Solid Edge part; units mm, degrees
sketch "Sketch1" plane through (0, 0, 0) normal (0, 0, 1) x (1, 0, 0)
  line L0 (-42.5, -23) -> (42.5, -23)
  line L1 (42.5, -23) -> (42.5, 23)
  line L2 (42.5, 23) -> (-42.5, 23)
  line L3 (-42.5, 23) -> (-42.5, -23)
  dimension "D1" = 42.5
  dimension "D2" = 42.5
extrude "Protrusion1" add sketch "Sketch1" along normal mid plane 27
sketch "Sketch2" plane through (0, 0, -13.5) normal (0, 0, -1) x (0, 1, 0)
  line L0 (-0.89, 32.61) -> (17.11, 32.61)
  line L1 (17.11, 32.61) -> (17.11, -22.39)
  line L2 (17.11, -22.39) -> (-0.89, -22.39)
  line L3 (-0.89, -22.39) -> (-0.89, 32.61)
extrude "Extrusionsausprägung_2" add sketch "Sketch2" along normal blind 4
sketch "Sketch3" plane through (0, 0, 13.5) normal (0, 0, 1) x (0, 1, 0)
  line L0 (23, -5.61) -> (23, 5.89)
  line L1 (23, 5.89) -> (21.29, 5.89)
  line L2 (21.29, 5.89) -> (21.29, 7.39)
  line L3 (21.29, 7.39) -> (16.29, 7.39)
  line L4 (16.29, 7.39) -> (16.29, 22.89)
  line L5 (16.29, 22.89) -> (2.29, 22.89)
  line L6 (2.29, 22.89) -> (2.29, 14.39)
  line L7 (2.29, 14.39) -> (-9.29, 14.39)
  line L8 (-9.29, 14.39) -> (-16.29, 7.39)
  line L9 (-21.29, 7.39) -> (-16.29, 7.39)
  line L10 (-21.29, 5.89) -> (-21.29, 7.39)
  line L11 (-23, 5.89) -> (-21.29, 5.89)
  line L12 (-23, -5.61) -> (-23, 5.89)
  dimension "D1" = 21.29
  dimension "D2" = 16.29
revolve "RevolvedCutout1" cut sketch "Sketch3" angle 360 about axis through (5.61, -23, 13.5) along (0, 1, 0)
sketch "Sketch4" plane through (-24.195, 0, 13.5) normal (0, 0, 1) x (1, 0, 0)
  line L0 (-5.355, 12) -> (-0.255, 12)
  line L1 (-0.255, 0) -> (-0.255, 12)
  line L2 (-5.355, 0) -> (-0.255, 0)
  line L3 (-5.355, 12) -> (-5.355, 0)
  dimension "D1" = 5.355
revolve "RevolvedCutout2" cut sketch "Sketch4" angle 360 about axis through (0, 0, 13.5) along (1, 0, 0)
sketch "Sketch5" plane through (-24.195, 0, 13.5) normal (0, 0, 1) x (1, 0, 0)
  line L0 (-0.255, 10.5) -> (3.745, 10.5)
  line L1 (3.745, 10.5) -> (12.745, 7.5)
  line L2 (12.745, 7.5) -> (12.745, 0)
  line L3 (-0.255, 0) -> (12.745, 0)
  line L4 (-0.255, 10.5) -> (-0.255, 0)
  dimension "D1" = 0.255
revolve "RevolvedCutout3" cut sketch "Sketch5" angle 360 about axis through (-42.5, 0, 13.5) along (1, 0, 0)
sketch "Sketch6" plane through (-24.195, 0, 13.5) normal (0, 0, 1) x (1, 0, 0)
  line L0 (-18.305, 0) -> (-5.355, 0)
  line L1 (-5.355, 0) -> (-5.355, -10.5)
  line L2 (-5.355, -10.5) -> (-18.305, -10.5)
  line L3 (-18.305, -10.5) -> (-18.305, 0)
revolve "RevolvedCutout4" cut sketch "Sketch6" angle 360 about axis through (0, 0, 13.5) along (1, 0, 0)
hole "Bohrung_1" at (38.1, 18.6, 13.5) direction (0, 0, -1) diameter 5.8 end up to next
hole "Hole1" at (38.1, -18.6, 13.5) direction (0, 0, -1) diameter 5.8 end up to next
hole "Hole2" at (-33.1, -18.6, 13.5) direction (0, 0, -1) diameter 5.8 end up to next
hole "Hole3" at (-33.1, 18.6, 13.5) direction (0, 0, -1) diameter 5.8 end up to next
properties material "Polykarbonat"
Part model, mm, in its own coordinate system. A direction names the side the tool comes from. Round coordinates to 2 decimals unless told otherwise and drop trailing zeros. Write each loop counter-clockwise with the first axis right and the second up, starting at its lowest first coordinate (ties: lowest second). Pieces come first, ordered by that corner, then holes. Notation, with made-up numbers: (-25.75, 3) -> (-3.75, 3) arc R11 cw to (-3.75, 12) -> close; hole circle Ø2 at (-40, 79.5). An arc over 180 degrees is marked (long way). Return JSON: item names as keys, results as strings. Group by question number.
Q1. Saw through at B-B on x = -33.1. Write the cut outline in (y, z), plus the area to 3 significant figures.
Q2. Saw through at D-D on z = -12.5. Write the cut outline in (x, y), plus the area to 3 significant figures.
Q3. Probe L1, parallel to Y at x = -33.1, z = -2.5; L2, parallel to Y at x = -3.5, z = -5; L3, parallel to Y at x = -34.5, z = -13. List the from-to ranges inside material, lowest first. Write a range as [from, to].
Q4. Saw through at A-A on y = 18.6. Write the cut outline in (x, z).
Q5. Pin check, flat tips, straight feed: pin 1 (4.5 mm diameter, centred on y = 6.5, z = -16, fed in from +X); pin 2 (2 mm diameter, centred on y = 8, z = -16, fed in from -X); pin 3 (6.5 mm diameter, centred on x = -33.1, y = -18.6, fed in from -Z). Stop position of each tip, or through.
Q6. Saw through at C-C on x = 5.61. Write the cut outline in (y, z).
Q7. Which spindle directions (+Z, -Z, +X, -X, +Y, -Y) get a long thin tool onto all of the face, cutting with end or side? Do faces 5 (the flat face through (42.5, 0, 0)), 6 (the flat face through (5.7, 21.29, 1.7)), 7 (the cylindrical face through (-22.866, -3.807, 3.715)), 8 (the flat face through (5, 17.11, -15)). Say none if no direction does.
Q8. Mould opens along Y. For faces 1 (the flat face through (32, 0, 13.5)), 2 (the conical face through (5.905, -15.852, 0.065)), 3 (the cylindrical face through (-36, 0, 3)), 4 (the flat face through (5, -0.89, -15)) say: pulls with the +Y half, pulls with the -Y half, needs draft (parallel to the pull), parting line crosses it, or undercut.
Answer:
{
 "1": {"outline": "(-23, -13.5) -> (-21.5, -13.5) -> (-21.5, 13.5) -> (-23, 13.5) -> close; (-15.7, -13.5) -> (15.7, -13.5) -> (15.7, 13.5) -> (10.5, 13.5) arc R10.5 cw to (-10.5, 13.5) -> (-15.7, 13.5) -> close; (21.5, -13.5) -> (23, -13.5) -> (23, 13.5) -> (21.5, 13.5) -> close", "area": "756 mm2"},
 "2": {"outline": "(-42.5, -23) -> (42.5, -23) -> (42.5, 23) -> (-42.5, 23) -> close; hole circle Ø5.8 at (-33.1, -18.6); hole circle Ø5.8 at (-33.1, 18.6); hole (-6.06, 2.29) -> (17.28, 2.29) -> (17.28, 16.29) -> (-6.06, 16.29) -> close; hole circle Ø5.8 at (38.1, -18.6); hole circle Ø5.8 at (38.1, 18.6)", "area": "3,480 mm2"},
 "3": {"L1": "[-23, -21.5], [-15.7, 15.7], [21.5, 23]", "L2": "[-23, 2.29], [16.29, 23]", "L3": "[-23, -21.14], [-16.06, 16.06], [21.14, 23]"},
 "4": {"outline": "(-42.5, -13.5) -> (-36, -13.5) -> (-36, 13.5) -> (-42.5, 13.5) -> close; (-30.2, -13.5) -> (35.2, -13.5) -> (35.2, 13.5) -> (18.61, 13.5) arc R13 cw to (-7.39, 13.5) -> (-30.2, 13.5) -> close; (41, -13.5) -> (42.5, -13.5) -> (42.5, 13.5) -> (41, 13.5) -> close"},
 "5": {"pin 1": "x = 32.61", "pin 2": "x = -22.39", "pin 3": "z = -13.5"},
 "6": {"outline": "(-23, -13.5) -> (-0.89, -13.5) -> (-0.89, -17.5) -> (17.11, -17.5) -> (17.11, -13.5) -> (23, -13.5) -> (23, 2) -> (21.29, 2) -> (21.29, 0.5) -> (16.29, 0.5) -> (16.29, -15) -> (2.29, -15) -> (2.29, -6.5) -> (-9.29, -6.5) -> (-16.29, 0.5) -> (-21.29, 0.5) -> (-21.29, 2) -> (-23, 2) -> close"},
 "7": {"face 5": "+Z, -Z, +X, +Y, -Y", "face 6": "+Z", "face 7": "+Z, -X", "face 8": "-Z, +X, -X, +Y"},
 "8": {"face 1": "needs draft", "face 2": "undercut", "face 3": "undercut", "face 4": "pulls with the -Y half"}
}
